Part model, mm, in its own coordinate system. Face numbers are marked on the shaded views. A direction names the side the tool comes from. Coordinates: 2 decimals unless noted, no trailing zeros. Loops run counter-clockwise (first coordinate to the right, second up) from the corner with the lowest first, then second, coordinate; pieces in that order, holes last. Notation, with made-up numbers: M 49,10.25 L 83,10.25 A23 cw 83,43.25 Z; hole C -6,-9 d9. An arc over 180 degrees is marked long. Use a Markdown table: item, result. Add a question column.
1) Band-saw the part on A-A (y = 80.5). List the corners of the cut face in (x, z).
2) Band-saw the part on D-D (z = 21). List the corners of the cut face in (x, y).
3) Pin check, flat tips, straight feed: pin 1 Ø2 at (x, z) = (133, 49.5) entering from -Y; pin 2 Ø10 at (x, y) = (-140, -2) entering from +Z; pin 3 Ø14.5 at (x, y) = (-174.5, -87) entering from +Z. Stop position of each tip, or through.
4) Wall check: probe 1 along X at (y, z) = (17, 56); probe 2 along X at (y, z) = (-62.5, 6); probe 3 along Y at (x, z) = (-127, 64). Give the ranges that are in metal, low to high. Write a range as from..to.
5) Band-saw the part on C-C (x = 72). List the corners of the cut face in (y, z).
6) Pull direction Y, two halves, no side cores. Call the marked faces 3, 4 and 5: released by +Y, released by -Y, zero draft, split by the parting line, or undercut.
7) Tool access for the marked faces 1 and 2: list every direction of +Z, -Z, +X, -X, +Y, -Y with a clear straight run to the whole face (end or side of a thin tool).
8) Band-saw the part on B-B (z = 83.5). List the corners of the cut face in (x, y).
from build123d import *

# Parameters (mm, degrees)
F0_W     = 385.718018
F0_H     = 222.336978
F1_DEPTH = 89.263966
F2_T     = -2.54
F3_W     = 385.718018
F3_H     = 89.263966
F4_DEPTH = 8.865619
F5_W     = 29.299758
F5_H     = 44.448814
F6_DEPTH = 25.4


with BuildPart() as f1:
    # F0 (on Top) → F1 (new body)
    with BuildSketch(Plane.XY):
        Rectangle(F0_W, F0_H)
    extrude(amount=F1_DEPTH)

    # F2
    f2_openings = [f1.faces().sort_by_distance(p)[0] for p in [
        (0, 0, 89.263966),
    ]]
    offset(amount=F2_T, openings=f2_openings)

    # F3 (on face) → F4 (cut)
    with BuildSketch(Plane.XZ.offset(111.168489)):
        with Locations((0, 44.631983)):
            Rectangle(F3_W, F3_H)
    extrude(amount=-F4_DEPTH, mode=Mode.SUBTRACT)

    # F5 (on face) → F6 (join)
    with BuildSketch(Plane.XY.offset(2.54)):
        with Locations((-175.66913, -80.078463)):
            Rectangle(F5_W, F5_H)
    extrude(amount=F6_DEPTH)


solid = f1.part
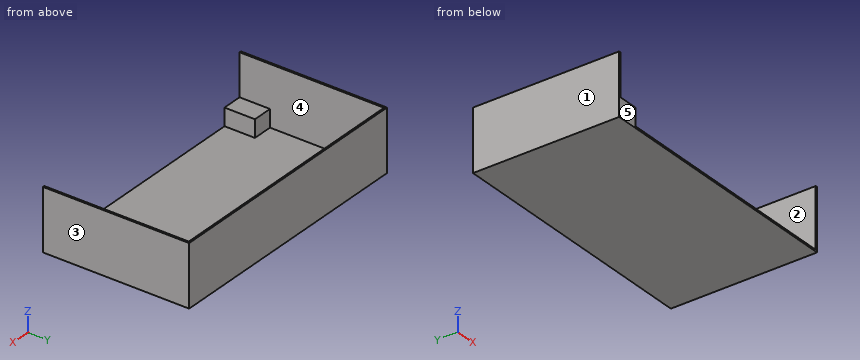
Entries:
| question | item | result |
|---|---|---|
| 1 | outline | M -192.86,0 L 192.86,0 L 192.86,89.26 L 190.32,89.26 L 190.32,2.54 L -190.32,2.54 L -190.32,89.26 L -192.86,89.26 Z |
| 2 | outline | M -192.86,-102.3 L -161.02,-102.3 L -161.02,-57.85 L -190.32,-57.85 L -190.32,108.63 L 190.32,108.63 L 190.32,-102.3 L 192.86,-102.3 L 192.86,111.17 L -192.86,111.17 Z |
| 3 | pin 1 | y = 108.63 |
| 3 | pin 2 | z = 2.54 |
| 3 | pin 3 | z = 27.94 |
| 4 | probe 1 | -192.86..-190.32, 190.32..192.86 |
| 4 | probe 2 | -192.86..-161.02, 190.32..192.86 |
| 4 | probe 3 | 108.63..111.17 |
| 5 | outline | M -102.3,0 L 111.17,0 L 111.17,89.26 L 108.63,89.26 L 108.63,2.54 L -102.3,2.54 Z |
| 6 | face 3 | zero draft |
| 6 | face 4 | undercut |
| 6 | face 5 | released by -Y |
| 7 | face 1 | +Z, -Z, -X, +Y, -Y |
| 7 | face 2 | +Z, -Y |
| 8 | outline | M -192.86,-102.3 L -190.32,-102.3 L -190.32,108.63 L 190.32,108.63 L 190.32,-102.3 L 192.86,-102.3 L 192.86,111.17 L -192.86,111.17 Z |
